Geometry: see drawing. Coordinates: mm, zero at the bounding-box minimum. Coordinates: 2 decimals unless noted, no trailing zeros. Order: outer loops, then holes, each group sorted by start corner. A loop starts at its lowest first (then second) coordinate and runs counter-clockwise, first axis right, second up. Notation, with made-up numbers: M 32.5,9 L 56.5,9 A24 cw 56.5,32 Z; hole C 1,-34 d10. An arc over 180 degrees is marked long. One line per item, written item: value.
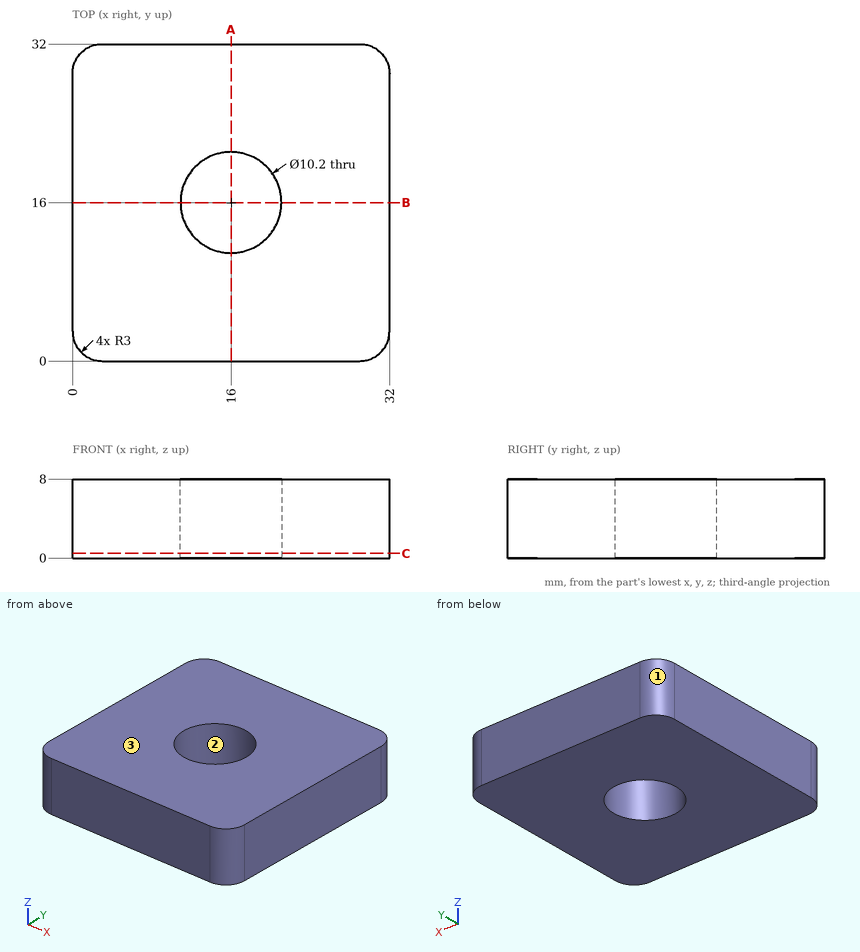
(1) Draft query along X for the marked faces 1, 2 and 3. Return one class per face: released by +X, released by -X, zero draft, split by the parting line, or undercut.
Data:
face 1: released by -X
face 2: undercut
face 3: zero draft
(2) Cut plane C-C on z = 0.5. Output: boundary loops of the cut face in (x, y).
Data:
outline: M 0,3 A3 ccw 3,0 L 29,0 A3 ccw 32,3 L 32,29 A3 ccw 29,32 L 3,32 A3 ccw 0,29 Z; hole C 16,16 d10.2
(3) Cut plane A-A on x = 16. Output: boundary loops of the cut face in (y, z), plus the area to 3 significant figures.
Data:
outline: M 0,0 L 10.9,0 L 10.9,8 L 0,8 Z; M 21.1,0 L 32,0 L 32,8 L 21.1,8 Z
area: 174 mm2
(4) Ray query, line 1 (Y direction, x = 16, z = 5.75); line 2 (Y direction, x = 13.5, z = 7); line 3 (X direction, y = 18, z = 6.5). Return the intervals inside material, ascending. Write a range as from..to.
Data:
line 1: y = 0..10.9, 21.1..32
line 2: y = 0..11.55, 20.45..32
line 3: x = 0..11.31, 20.69..32
(5) First-contact query: pin 1 (9 mm diameter, centred on x = 16, y = 16, fed in from -Z). Flat tip, straight axial feed; report the tip coordinate or a pass-through.
Data:
pin 1: passes through
